Autodesk Inventor part; units mm, degrees
ref_plane "YZ Plane" through (0, 0, 0) normal (1, 0, 0) x (0, 1, 0)
ref_plane "XZ Plane" through (0, 0, 0) normal (0, 1, 0) x (-1, 0, 0)
sketch "Sketch1" plane through (0, 0, 0) normal (0, 1, 0) x (-1, 0, 0)
  line L0 (0, 0) -> (21.668, 0)
  line L1 (21.668, 0) -> (21.668, -61.4)
  line L2 (21.668, -61.4) -> (0, -61.4)
  line L3 (0, -61.4) -> (0, 0)
  dimension "d0" = 21.668
  dimension "d1" = 61.4
extrude "Extrusion1" add sketch "Sketch1" along normal blind 83
sketch "Sketch2" plane through (0, 83, 0) normal (0, 1, 0) x (1, 0, 0)
  line L0 (0, 0) -> (0, 1.4)
  line L1 (0, 0) -> (0, 61.4)
  line L2 (0, 1.4) -> (-20.268, 1.4)
  line L3 (-21.668, 61.4) -> (-21.668, 0)
  line L4 (-20.268, 1.4) -> (-20.268, 61.4)
  line L5 (0, 61.4) -> (-21.668, 61.4)
  line L6 (-20.268, 61.4) -> (0, 61.4)
  line L7 (0, 61.4) -> (0, 1.4)
  line L8 (-21.668, 61.4) -> (0, 61.4)
  line L9 (0, 61.4) -> (0, 62.8)
  line L10 (0, 62.8) -> (-21.668, 62.8)
  line L11 (-21.668, 62.8) -> (-21.668, 61.4)
  dimension "d4" = 1.4
  dimension "d5" = 20.268
  dimension "d6" = 1.4
extrude "Extrusion2" add sketch "Sketch2" against normal blind 83 contours L5 L11 L10 L9
sketch "Sketch3" plane through (0, 83, 0) normal (0, 1, 0) x (1, 0, 0)
  line L0 (0, 0) -> (0, 62.8)
  line L1 (0, 0) -> (0, 1.4)
  line L2 (0, 1.4) -> (-20.268, 1.4)
  line L3 (-20.268, 1.4) -> (-20.268, 61.4)
  line L4 (-21.668, 62.8) -> (-21.668, 0)
  line L5 (-20.268, 61.4) -> (0, 61.4)
  dimension "d9" = 1.4
  dimension "d10" = 20.268
  dimension "d11" = 60
extrude "Extrusion3" cut sketch "Sketch3" against normal blind 129.5
sketch "Sketch4" plane through (0, 83, 0) normal (0, 1, 0) x (1, 0, 0)
  line L0 (0, 0) -> (0, 1.4)
  line L1 (0, 0) -> (0, -2)
  line L2 (0, -2) -> (-3.619, -2)
  line L3 (-20.268, 1.4) -> (0, 1.4)
  line L4 (-3.619, -2) -> (-3.619, 0)
  line L5 (-21.668, 0) -> (0, 0)
  line L6 (-3.619, 0) -> (-7.238, 0)
  line L7 (-7.238, 0) -> (-7.238, 1.4)
  line L8 (-7.238, 1.4) -> (-7.238, 4.4)
  line L9 (-7.238, 4.4) -> (-9.238, 4.4)
  line L10 (-9.238, 4.4) -> (-9.238, 2.9)
  line L11 (-9.238, 2.9) -> (-10.738, 2.9)
  line L12 (-10.738, 2.9) -> (-10.738, 4.4)
  line L13 (-10.738, 4.4) -> (-12.738, 4.4)
  line L14 (-12.738, 4.4) -> (-12.738, 1.4)
  dimension "d14" = 2
  dimension "d15" = 3.619
  dimension "d16" = 3.619
  dimension "d17" = 3
  dimension "d18" = 2
  dimension "d19" = 1.5
  dimension "d20" = 1.5
  dimension "d21" = 2
extrude "Extrusion4" add sketch "Sketch4" against normal blind 83 contours L3 L14 L13 L12 L11 L10 L9 L8 | L1 L2 L4 L5
ref_plane "Work Plane1" through (0, 0, -31.4) normal (0, 0, 1) x (1, 0, 0)
mirror "Mirror1" about plane through (0, 0, -31.4) normal (0, 0, 1) of "Extrusion4"
sketch "Sketch5" plane through (-21.668, 0, 0) normal (-1, 0, 0) x (0, 0, 1)
  line L0 (-62.8, 83) -> (-62.8, 0)
  line L1 (0, 0) -> (-62.8, 0)
  line L2 (-62.8, 0) -> (-62.8, 83)
  line L3 (-62.8, 83) -> (0, 83)
  line L4 (0, 83) -> (0, 0)
extrude "Extrusion5" cut sketch "Sketch5" against normal blind 6.454
sketch "Sketch6" plane through (-15.214, 0, 0) normal (-1, 0, 0) x (0, 0, 1)
  line L0 (2, 0) -> (0, 0)
  line L1 (-62.8, 83) -> (-61.4, 83)
  line L2 (0, 0) -> (-62.8, 0)
  line L3 (-62.8, 0) -> (-62.8, 83)
  line L4 (-62.8, 83) -> (0, 83)
  line L5 (0, 83) -> (0, 0)
extrude "Extrusion6" add sketch "Sketch6" along normal blind 1.4
properties part number "kabza başlık"
Design review of the part built by this model. Coordinates are the model's own, in mm. A direction names the side the tool comes from. Coordinates: 2 decimals unless noted, no trailing zeros. Order: outer loops, then holes, each group sorted by start corner. A loop starts at its lowest first (then second) coordinate and runs counter-clockwise, first axis right, second up.
Item 1: Take a section at C-C, the plane z = -42. Write out the cut boundary in (x, y).
Item 2: The part is to be moulded in two halves that separate along X. For faces 6 (the flat face through (-16, 83, -32)), 7 (the flat face through (-14, 42, -1.4)), 8 (the flat face through (-16.614, 42, -32)), say which applies: pulls with the +X half, pulls with the -X half, needs draft (parallel to the pull), parting line crosses it, or undercut.
Item 3: Take a section at B-B, the plane y = 39. Write out the cut boundary in (x, z).
Item 4: Take a section at A-A, the plane x = -8.25. Write out the cut boundary in (y, z).
Item 5: For line 1 (X direction, y = 3, z = -4); line 2 (Z direction, x = -6.75, y = 49.5); line 3 (Z direction, x = -3, y = 68), list the stretches that pass through material, from the lowest coordinate up.
Item 6: For pin 1 Ø1.5 at (y, z) = (56.5, -51.5) entering from +X; pin 2 Ø0.6 at (x, y) = (-12, 21) entering from -Z; pin 3 Ø1 at (y, z) = (59, 1) entering from -X, all flat-tipped, find the tip position at first contact; note any pin that passes through.
Item 7: For faces 1 (the flat face through (-7.238, 42, -3)), 2 (the flat face through (-10, 41, -62.8)), 3 (the flat face through (-12.738, 42, -3)), 4 (the flat face through (-3.619, 42, 1)), 5 (the flat face through (0, 41, 0)), list the 3-axis set-ups (+Z, -Z, +X, -X, +Y, -Y) from which the entire face can be reached by the end or side of a thin tool; tool diameter is ignored.
The answers:
1. outline: (-16.61, 0) - (-15.21, 0) - (-15.21, 83) - (-16.61, 83) - close
2. face 6: needs draft
2. face 7: undercut
2. face 8: pulls with the -X half
3. outline: (-16.61, -62.8) - (-3.62, -62.8) - (-3.62, -64.8) - (0, -64.8) - (0, -61.4) - (-7.24, -61.4) - (-7.24, -58.4) - (-9.24, -58.4) - (-9.24, -59.9) - (-10.74, -59.9) - (-10.74, -58.4) - (-12.74, -58.4) - (-12.74, -61.4) - (-15.21, -61.4) - (-15.21, -1.4) - (-12.74, -1.4) - (-12.74, -4.4) - (-10.74, -4.4) - (-10.74, -2.9) - (-9.24, -2.9) - (-9.24, -4.4) - (-7.24, -4.4) - (-7.24, -1.4) - (0, -1.4) - (0, 2) - (-3.62, 2) - (-3.62, 0) - (-16.61, 0) - close
4. outline: (0, -62.8) - (83, -62.8) - (83, -58.4) - (0, -58.4) - close; (0, -4.4) - (83, -4.4) - (83, 0) - (0, 0) - close
5. line 1: x = -16.61 to -15.21, -12.74 to -10.74, -9.24 to -7.24
5. line 2: z = -62.8 to -61.4, -1.4 to 0
5. line 3: z = -64.8 to -61.4, -1.4 to 2
6. pin 1: stops at x = -15.21
6. pin 2: stops at z = -62.8
6. pin 3: stops at x = -3.62
7. face 1: +X, +Y, -Y
7. face 2: -Z, -X, +Y, -Y
7. face 3: +Y, -Y
7. face 4: +Z, -X, +Y, -Y
7. face 5: +Z, -Z, +X, +Y, -Y
